```python
from build123d import *

# Parameters (mm, degrees)
SKETCH_1_W          = 34
SKETCH_1_H          = 30
SKETCH_1_R          = 5.25
EXTRUDE_1_DEPTH     = 30
SKETCH_2_R          = 1.75
CUT_EXTRUDE_1_DEPTH = 10
SKETCH_4_R          = 2
CUT_EXTRUDE_3_DEPTH = 10


with BuildPart() as part:
    # 草图1 → 凸台-拉伸1 (new body)
    with BuildSketch(Plane.XY):
        Rectangle(SKETCH_1_W, SKETCH_1_H)
        Circle(SKETCH_1_R, mode=Mode.SUBTRACT)
    extrude(amount=EXTRUDE_1_DEPTH)

    # 草图2 → 切除-拉伸1 (cut)
    with BuildSketch(Plane.XY.offset(30)):
        with Locations((-8, 0)):
            Circle(SKETCH_2_R)
        with Locations((0, 8)):
            Circle(SKETCH_2_R)
        with Locations((8, 0)):
            Circle(SKETCH_2_R)
        with Locations((0, -8)):
            Circle(SKETCH_2_R)
    extrude(amount=-CUT_EXTRUDE_1_DEPTH, mode=Mode.SUBTRACT)

    # 草图4 → 切除-拉伸3 (cut)
    with BuildSketch(Plane(origin=(0, 15, 0), x_dir=(1, 0, 0), z_dir=(0, 1, 0))):
        with Locations(Location((12, -25, 0), (0, 0, 180))):
            Circle(SKETCH_4_R)
        with Locations(Location((-12, -25, 0), (0, 0, 180))):
            Circle(SKETCH_4_R)
        with Locations(Location((-12, -5, 0), (0, 0, 180))):
            Circle(SKETCH_4_R)
        with Locations(Location((12, -5, 0), (0, 0, 180))):
            Circle(SKETCH_4_R)
    extrude(amount=-CUT_EXTRUDE_3_DEPTH, mode=Mode.SUBTRACT)


solid = part.part
```
Design review of the part built by this model. Coordinates are the model's own, in mm. A direction names the side the tool comes from. Coordinates: 2 decimals unless noted, no trailing zeros. Order: outer loops, then holes, each group sorted by start corner. A loop starts at its lowest first (then second) coordinate and runs counter-clockwise, first axis right, second up. Notation, with made-up numbers: (18, 45) - (22, 45) arc R20 ccw to (22, 54) - close; hole circle Ø7 at (38, 61.25). An arc over 180 degrees is marked (long way). One line per question, with ' | ' between items.
Q1. Clearance check with flat-ended pins moving along their axes: pin 1 Ø3 at (x, y) = (-8, 0) entering from +Z; pin 2 Ø1.2 at (x, z) = (-12.5, 5) entering from +Y; pin 3 Ø5.5 at (x, y) = (-8, 0) entering from +Z. State where each tip first meets the part, or that it passes through.
Answer key:
pin 1: stops at z = 20 | pin 2: stops at y = 5 | pin 3: stops at z = 30
Q2. For faces 1 (the flat face through (12, 5, 5)), 2 (the cylindrical face through (1.617, -8.67, 25.07)), 3 (the flat face through (-4, 4, 0)), list the 3-axis set-ups (+Z, -Z, +X, -X, +Y, -Y) from which the entire face can be reached by the end or side of a thin tool; tool diameter is ignored.
Answer key:
face 1: +Y | face 2: +Z | face 3: -Z, +X, -X, +Y, -Y
Q3. Consider section D-D, the plane y = 0. Give the boundary of the cut face in (x, z).
Answer key:
outline: (-17, 0) - (-5.25, 0) - (-5.25, 30) - (-6.25, 30) - (-6.25, 20) - (-9.75, 20) - (-9.75, 30) - (-17, 30) - close; (5.25, 0) - (17, 0) - (17, 30) - (9.75, 30) - (9.75, 20) - (6.25, 20) - (6.25, 30) - (5.25, 30) - close
Q4. The part is to be moulded in two halves that separate along Y. For faces 4 (the cylindrical face through (13.6, 10.1, 23.8)), 5 (the cylindrical face through (-0.228, 9.735, 25.07)), 6 (the flat face through (-12, 5, 25)), say which applies: +Y half, -Y half, draft (parallel to the pull), parting line (faces both ways), or undercut.
Answer key:
face 4: draft | face 5: undercut | face 6: +Y half
Q5. To check wall thickness, follow line 1 along Z through (x, y) = (-12, 8.75); line 2 along Y through (x, z) = (-8, 28.25); line 3 along Y through (x, z) = (-1.5, 28.25). State the ranges of each line that lie inside material, in increasing order.
Answer key:
line 1: z = 0 to 3, 7 to 23, 27 to 30 | line 2: y = -15 to -1.75, 1.75 to 15 | line 3: y = -15 to -8.9, -7.1 to -5.03, 5.03 to 7.1, 8.9 to 15
Q6. Consider section B-B, the plane x = 0. Give the boundary of the cut face in (y, z).
Answer key:
outline: (-15, 0) - (-5.25, 0) - (-5.25, 30) - (-6.25, 30) - (-6.25, 20) - (-9.75, 20) - (-9.75, 30) - (-15, 30) - close; (5.25, 0) - (15, 0) - (15, 30) - (9.75, 30) - (9.75, 20) - (6.25, 20) - (6.25, 30) - (5.25, 30) - close
Q7. Consider section A-A, the plane y = 10.25. Give the boundary of the cut face in (x, z), then the cut area to 3 significant figures.
Answer key:
outline: (-17, 0) - (17, 0) - (17, 30) - (-17, 30) - close; hole circle Ø4 at (-12, 5); hole circle Ø4 at (-12, 25); hole circle Ø4 at (12, 5); hole circle Ø4 at (12, 25) | area: 970 mm2
Q8. Consider section C-C, the plane z = 5. Give the boundary of the cut face in (x, y).
Answer key:
outline: (-17, -15) - (17, -15) - (17, 15) - (14, 15) - (14, 5) - (10, 5) - (10, 15) - (-10, 15) - (-10, 5) - (-14, 5) - (-14, 15) - (-17, 15) - close; hole circle Ø10.5 at (0, 0)
